For this review, take the finished solid that the model builds, in its own axes (mm). Give positions to 0.01 mm unless a question says otherwise; leave off trailing zeros. Order: outer loops, then holes, each group sorted by start corner. A loop starts at its lowest first (then second) coordinate and runs counter-clockwise, first axis right, second up.
from build123d import *


with BuildPart() as part:
    # Esquisse1 → Révolution1 (revolve)
    with BuildSketch(Plane.XY):
        with BuildLine():
            Line((-1.497157288, -0.117157288), (-1.397157288, -0.217157288))
            ThreePointArc((-1.397157288, -0.217157288), (-1.310448187, -0.346926627), (-1.28, -0.5))
            Line((-1.28, -0.5), (-1.28, -5.2))
            Line((-1.28, -5.2), (-1.48, -5.2))
            Line((-1.48, -5.2), (-1.48, -0.5))
            ThreePointArc((-1.48, -0.5), (-1.495224093, -0.423463314), (-1.538578644, -0.358578644))
            Line((-1.538578644, -0.358578644), (-1.638578644, -0.258578644))
            ThreePointArc((-1.638578644, -0.258578644), (-1.703463314, -0.215224093), (-1.78, -0.2))
            Line((-1.78, -0.2), (-1.825735931, -0.2))
            ThreePointArc((-1.825735931, -0.2), (-1.902272618, -0.215224093), (-1.967157288, -0.258578644))
            Line((-1.967157288, -0.258578644), (-2.108578644, -0.4))
            Line((-2.108578644, -0.4), (-2.25, -0.258578644))
            Line((-2.25, -0.258578644), (-2.108578644, -0.117157288))
            ThreePointArc((-2.108578644, -0.117157288), (-1.978809304, -0.030448187), (-1.825735931, 0))
            Line((-1.825735931, 0), (-1.78, 0))
            ThreePointArc((-1.78, 0), (-1.626926627, -0.030448187), (-1.497157288, -0.117157288))
        make_face()
    revolve(axis=Axis((0, 0, 0), (0, -1, 0)))


solid = part.part
1) To check wall thickness, follow line 1 (X direction, y = -1.55, z = 0); line 2 (Y direction, x = -1.6, z = -0.9). State the ranges of each line that lie inside material, in increasing order.
Answer sheet:
line 1: x = -1.48 to -1.28, 1.28 to 1.48
line 2: y = -0.2 to 0
2) Draft analysis for pull direction X (two halves, no side actions). For faces 1 (the face through (1.28, -2.88, -0.06)), 2 (the face through (1.174, -2.817, 0.901)), state which applies: +X half, -X half, draft (parallel to the pull), parting line (faces both ways), or undercut.
Answer sheet:
face 1: undercut
face 2: parting line
3) We need section C-C on y = -4.8. Give the boundary of the cut face in (x, z).
Answer sheet:
outline: circle Ø2.96 at (0, 0); hole circle Ø2.56 at (0, 0)
4) Clearance check with flat-ended pins moving along their axes: pin 1 (1 mm diameter, centred on x = 1, y = -2.5, fed in from -Z); pin 2 (2 mm diameter, centred on x = 0, z = 1.5, fed in from -Y); pin 3 (2.5 mm diameter, centred on x = 0, z = 0, fed in from +Y). State where each tip first meets the part, or that it passes through.
Answer sheet:
pin 1: stops at z = -1.39
pin 2: stops at y = -5.2
pin 3: passes through
